Here's how the part is built. I have some questions about the finished solid (model axes, mm). A direction names the side the tool comes from. Give positions to 0.01 mm unless a question says otherwise; leave off trailing zeros. Write each loop counter-clockwise with the first axis right and the second up, starting at its lowest first coordinate (ties: lowest second). Pieces come first, ordered by that corner, then holes. Notation, with made-up numbers: M -6,-4.5 L 43,-4.5 A23 cw 43,14.5 Z; hole C 7,-34 d10. An arc over 180 degrees is marked long. Answer as CSV lines item,"result". Start each with the question number.
Q1. Suppose I cut it at A-A (z = 7). Write out the boundary of the cut face in (x, y).
Q2. For pin 1 (1.6 mm diameter, centred on x = -80, y = -20, fed in from +Z); pin 2 (0.8 mm diameter, centred on y = -19.5, z = 25, fed in from +X); pin 3 (0.8 mm diameter, centred on x = -80, y = -19.5, fed in from -Z), each with a flat end and sliding along its axis, tell me the tip position at first contact or that it passes through.
Q3. Suppose I cut it at C-C (z = 57). Write out the boundary of the cut face in (x, y).
Q4. If I drill on line 1 along Y through (x, z) = (-94, 37); line 2 along X through (y, z) = (-18.9, 50); line 3 along X through (y, z) = (-17.1, 64), over which ranges is the centre line in solid material (lowest first)?
Q5. Suppose I cut it at B-B (x = -88). Write out the boundary of the cut face in (y, z).
Q6. On a 3-axis mill with a long thin cutter (end or side, diameter ignored), from which of +Z, -Z, +X, -X, +Y, -Y can I reach the whole of each face in a straight line? I mean faces 1 (the cylindrical face through (-92.696, -19.166, 63.324)), 2 (the cylindrical face through (-92.696, -19.166, 3.944)), 3 (the flat face through (-92, -17, 59.38)). Say none if no direction works.
Q7. Thinking about a two-plate mould opening in Z: for faces 4 (the flat face through (-152, -17, 59.38)), 5 (the flat face through (-125.5, -19.4, 0)), 6 (the flat face through (-125.2, -19.4, 67.38)), which applies, +Z half, -Z half, draft (parallel to the pull), parting line (faces both ways), or undercut?
```python
from build123d import *

# Parameters (mm, degrees)
SKETCH1_W             = 74.077377751
SKETCH1_H             = 1.5
BOSS_EXTRUDE1_DEPTH   = 67.38
SKETCH2_R             = 2
BOSS_EXTRUDE2_DEPTH   = 8
SKETCH3_R             = 0.769644957
SKETCH3_R_2           = 0.9
CUT_EXTRUDE1_DEPTH    = 8
BOSS_EXTRUDE3_START   = 8
SKETCH4_R             = 2
BOSS_EXTRUDE3_DEPTH   = 8
SKETCH5_R             = 0.9
SKETCH5_R_2           = 0.769644957
CUT_EXTRUDE2_DEPTH    = 8
BOSS_EXTRUDE4_START   = -20.367507575
BOSS_EXTRUDE4_DEPTH   = 1.5
BOSS_EXTRUDE4_START_2 = 64.08
BOSS_EXTRUDE4_2_DEPTH = 1.5
SKETCH7_W             = 5.986172604
SKETCH7_H             = 3.921086245
CUT_EXTRUDE4_DEPTH    = 174.349085042


with BuildPart() as part:
    # Sketch1 → Boss-Extrude1 (new body)
    with BuildSketch(Plane.XY):
        with Locations((-122.62921925, -19.617507575)):
            Rectangle(SKETCH1_W, SKETCH1_H)
    extrude(amount=BOSS_EXTRUDE1_DEPTH)

    # Sketch2 → Boss-Extrude2 (add)
    with BuildSketch(Plane.XY):
        with Locations((-151.644507933, -18.367507575)):
            Circle(SKETCH2_R)
        with Locations((-92.280362099, -18.367507575)):
            Circle(SKETCH2_R)
    extrude(amount=BOSS_EXTRUDE2_DEPTH)

    # Sketch3 → Cut-Extrude1 (cut)
    with BuildSketch(Plane(origin=(0, 0, 0), x_dir=(-1, 0, 0), z_dir=(0, 0, -1))):
        with Locations((151.644507933, -18.367507575)):
            Circle(SKETCH3_R)
        with Locations((92.280362099, -18.367507575)):
            Circle(SKETCH3_R_2)
    extrude(amount=-CUT_EXTRUDE1_DEPTH, mode=Mode.SUBTRACT)

    # Sketch4 → Boss-Extrude3 (add)
    with BuildSketch(Plane(origin=(0, 0, 67.38), x_dir=(-1, 0, 0), z_dir=(0, 0, -1)).offset(BOSS_EXTRUDE3_START)):
        with Locations((151.644507933, -18.367507575)):
            Circle(SKETCH4_R)
        with Locations((92.280362099, -18.367507575)):
            Circle(SKETCH4_R)
    extrude(amount=-BOSS_EXTRUDE3_DEPTH)

    # Sketch5 → Cut-Extrude2 (cut)
    with BuildSketch(Plane(origin=(0, 0, 59.38), x_dir=(-1, 0, 0), z_dir=(0, 0, -1))):
        with Locations((92.280362099, -18.367507575)):
            Circle(SKETCH5_R)
        with Locations((151.644507933, -18.367507575)):
            Circle(SKETCH5_R_2)
    extrude(amount=-CUT_EXTRUDE2_DEPTH, mode=Mode.SUBTRACT)

    # Boss-Extrude4: read off the stored shape, not the designer's step
    # Boss-Extrude4 outline → Boss-Extrude4 (add)
    with BuildSketch(Plane(origin=(0, 0, 0), x_dir=(1, 0, 0), z_dir=(0, 1, 0)).offset(BOSS_EXTRUDE4_START)):
        with BuildLine():
            ThreePointArc((-85.590530374, -66.08), (-85.004743937, -64.665786437), (-83.590530374, -64.08))
            Line((-83.590530374, -64.08), (-77.590530374, -64.08))
            ThreePointArc((-77.590530374, -64.08), (-76.176316812, -63.494213562), (-75.590530374, -62.08))
            Line((-75.590530374, -62.08), (-75.590530374, -56.08))
            ThreePointArc((-75.590530374, -56.08), (-76.176316812, -54.665786438), (-77.590530374, -54.08))
            Line((-77.590530374, -54.08), (-83.590530374, -54.08))
            ThreePointArc((-83.590530374, -54.08), (-85.004743937, -53.494213563), (-85.590530374, -52.08))
            Line((-85.590530374, -52.08), (-85.590530374, -66.08))
        make_face()
    extrude(amount=BOSS_EXTRUDE4_DEPTH)

    # Boss-Extrude4 2 outline → Boss-Extrude4 2 (add)
    with BuildSketch(Plane.XY.offset(BOSS_EXTRUDE4_START_2)):
        Polygon((-79.170711658, -18.867507575), (-82.010469997, -18.867507575), (-80.595461682, -19.68726796), align=None)
    extrude(amount=BOSS_EXTRUDE4_2_DEPTH)

    # Sketch7 → Cut-Extrude4 (cut, through all)
    with BuildSketch(Plane.XZ.offset(20.367507575)):
        with Locations((-80.502378911, 64.691696103)):
            Rectangle(SKETCH7_W, SKETCH7_H)
    extrude(amount=-CUT_EXTRUDE4_DEPTH, mode=Mode.SUBTRACT)


solid = part.part
```
Resolved:
1,outline,"M -159.67,-20.37 L -85.59,-20.37 L -85.59,-18.87 L -90.34,-18.87 A2 ccw long -94.22,-18.87 L -149.71,-18.87 A2 ccw long -153.58,-18.87 L -159.67,-18.87 Z; hole C -151.64,-18.37 d1.54; hole C -92.28,-18.37 d1.8"
2,pin 1,"z = 62.73"
2,pin 2,"x = -85.59"
2,pin 3,"z = 54.08"
3,outline,"M -159.67,-20.37 L -75.59,-20.37 L -75.59,-18.87 L -159.67,-18.87 Z"
4,line 1,"-20.37 to -18.87"
4,line 2,"-159.67 to -85.59"
4,line 3,"-153.19 to -150.1, -93.83 to -90.73"
5,outline,"M -20.37,0 L -18.87,0 L -18.87,67.38 L -20.37,67.38 Z"
6,face 1,"+Z"
6,face 2,"-Z"
6,face 3,"+X, -X, +Y"
7,face 4,"undercut"
7,face 5,"-Z half"
7,face 6,"+Z half"
